```python
from build123d import *

# Parameters (mm, degrees)
F1_DEPTH = 203.2
F2_R     = 1.905
F3_DEPTH = 31.751


with BuildPart() as f1:
    # F0 (on Right) → F1 (new body)
    with BuildSketch(Plane.YZ):
        Polygon((15.875, -14.605), (15.875, 15.875), (-15.875, 15.875), (-15.875, -14.605), (-14.605, -14.605), (-14.605, 14.605), (14.605, 14.605), (14.605, -14.605), align=None)
    extrude(amount=F1_DEPTH)

    # F2 (on face) → F3 (cut, through all)
    with BuildSketch(Plane.XZ.offset(15.875)):
        with Locations((15.875, 0)):
            Circle(F2_R)
        with Locations((23.495, 0)):
            Circle(F2_R)
    extrude(amount=-F3_DEPTH, mode=Mode.SUBTRACT)


solid = f1.part
```
Geometry: final body of the model. Coordinates: model frame, mm. A direction names the side the tool comes from. Round coordinates to 2 decimals unless told otherwise and drop trailing zeros. Write each loop counter-clockwise with the first axis right and the second up, starting at its lowest first coordinate (ties: lowest second). Pieces come first, ordered by that corner, then holes. Notation, with made-up numbers: M 70,15.25 L 129,15.25 A19 ccw 129,29.25 Z; hole C 83,28.25 d5. An arc over 180 degrees is marked long. Answer in a Markdown table with one row per item. Add a question column.
(1) Contact query for a flat-ended pin moving along its axis: pin 1 (3.5 mm diameter, centred on x = 23.495, z = 0, fed in from -Y). Output: stop coordinate, or through.
(2) Cut plane A-A, the plane z = 8.5. Return the cut outline in (x, y) (3 decimals), then the cut area to 3 significant figures.
(3) Cut plane C-C, the plane x = 96.5. Return the cut outline in (y, z) (3 decimals), then the cut area to 3 significant figures.
(4) Cut plane B-B, the plane z = 0. Return the cut outline in (x, y) (3 decimals), then the cut area to 3 significant figures.
(5) Cut plane D-D, the plane y = -11.5. Return the cut outline in (x, z) (3 decimals).
(6) Ray query, L1, parallel to Y at x = 118, z = 2.5 (3 decimals); L2, parallel to Z at x = 122, y = 9 (3 decimals). Return the intervals inside material, ascending.
(7) Reachability of faces 4 (the face through (100, -14.605, 0)), 5 (the face through (100, 15.875, 0)) from +Z, -Z, +X, -X, +Y, -Y: full face, straight path, thin tool, end or side. Return the list, or none.
(8) Draft query along Z for faces 1 (the face through (21.59, 15.23, 0.08)), 2 (the face through (100, -15.875, 1)), 3 (the face through (100, 0, 14.605)). Return one class per face: pulls with the +Z half, pulls with the -Z half, needs draft (parallel to the pull), parting line crosses it, or undercut.
Established:
| question | item | result |
|---|---|---|
| 1 | pin 1 | through |
| 2 | outline | M 0,-15.875 L 203.2,-15.875 L 203.2,-14.605 L 0,-14.605 Z; M 0,14.605 L 203.2,14.605 L 203.2,15.875 L 0,15.875 Z |
| 2 | area | 516 mm² |
| 3 | outline | M -15.875,-14.605 L -14.605,-14.605 L -14.605,14.605 L 14.605,14.605 L 14.605,-14.605 L 15.875,-14.605 L 15.875,15.875 L -15.875,15.875 Z |
| 3 | area | 115 mm² |
| 4 | outline | M 0,-15.875 L 13.97,-15.875 L 13.97,-14.605 L 0,-14.605 Z; M 0,14.605 L 13.97,14.605 L 13.97,15.875 L 0,15.875 Z; M 17.78,-15.875 L 21.59,-15.875 L 21.59,-14.605 L 17.78,-14.605 Z; M 17.78,14.605 L 21.59,14.605 L 21.59,15.875 L 17.78,15.875 Z; M 25.4,-15.875 L 203.2,-15.875 L 203.2,-14.605 L 25.4,-14.605 Z; M 25.4,14.605 L 203.2,14.605 L 203.2,15.875 L 25.4,15.875 Z |
| 4 | area | 497 mm² |
| 5 | outline | M 0,14.605 L 203.2,14.605 L 203.2,15.875 L 0,15.875 Z |
| 6 | L1 | -15.875 to -14.605, 14.605 to 15.875 |
| 6 | L2 | 14.605 to 15.875 |
| 7 | face 4 | -Z, +X, -X |
| 7 | face 5 | +Z, -Z, +X, -X, +Y |
| 8 | face 1 | undercut |
| 8 | face 2 | needs draft |
| 8 | face 3 | pulls with the -Z half |
